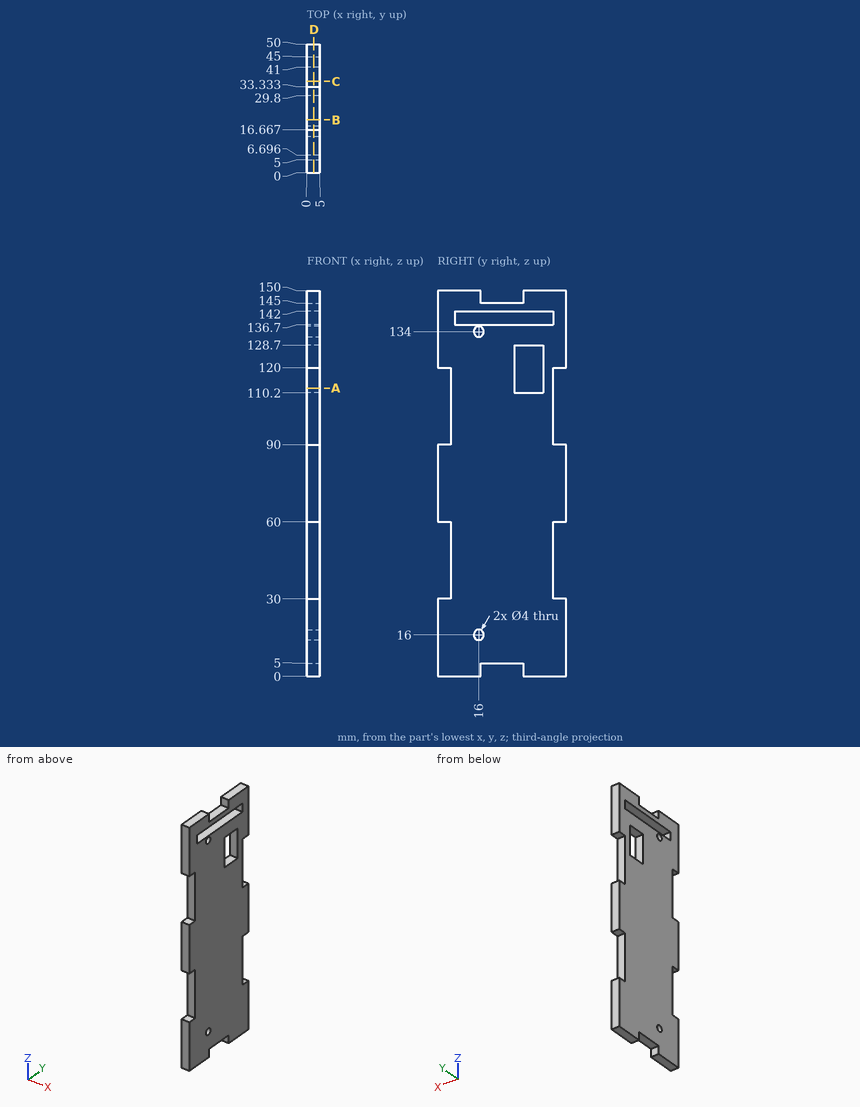
Answer from the drawing. Dimensions are ordinates in mm from the lowest x, y and z of the part. Round coordinates to 2 decimals unless told otherwise and drop trailing zeros. Write each loop counter-clockwise with the first axis right and the second up, starting at its lowest first coordinate (ties: lowest second). Pieces come first, ordered by that corner, then holes.
1. Straight lines are drawn through the part: L1, parallel to Z at x = 3.15, y = 47; L2, parallel to Z at x = 0.8, y = 31; L3, parallel to Y at x = 3.05, z = 134. For each, find the intervals that lie inside material, in ascending order.
2. The part is cut by section B-B, the plane y = 20.5. Determine the outline of the cut face in (x, z).
3. The part is cut by section D-D, the plane x = 2.7. State how many separate pieces and enclosed holes the cut face has, then the cut area to 3 significant figures.
4. Given pin 1 Ø5 at (y, z) = (23, 72) entering from -X; pin 2 Ø1.5 at (x, y) = (3.5, 23) entering from -Z; pin 3 Ø1.5 at (x, z) = (3.5, 50) entering from +Y, each flat-ended and moving along its own axis, determine where each tip first touches the part or whether it passes through.
5. The part is cut by section A-A, the plane z = 112. Determine the outline of the cut face in (x, y).
6. The part is cut by section C-C, the plane y = 35.5. Determine the outline of the cut face in (x, z).
Values:
1. L1: z = 0 to 30, 60 to 90, 120 to 150
1. L2: z = 5 to 110.2, 128.7 to 136.7, 142 to 145
1. L3: y = 0 to 14, 18 to 50
2. outline: (0, 5) - (5, 5) - (5, 136.7) - (0, 136.7) - close; (0, 142) - (5, 142) - (5, 145) - (0, 145) - close
3. separate pieces: 1
3. enclosed holes: 4
3. area: 6,300 mm2
4. pin 1: stops at x = 0
4. pin 2: stops at z = 5
4. pin 3: stops at y = 45
5. outline: (0, 5) - (5, 5) - (5, 29.8) - (0, 29.8) - close; (0, 41) - (5, 41) - (5, 45) - (0, 45) - close
6. outline: (0, 0) - (5, 0) - (5, 110.2) - (0, 110.2) - close; (0, 128.7) - (5, 128.7) - (5, 136.7) - (0, 136.7) - close; (0, 142) - (5, 142) - (5, 150) - (0, 150) - close
